Autodesk Inventor part; units mm, degrees
ref_plane "YZ Plane" through (0, 0, 0) normal (1, 0, 0) x (0, 1, 0)
ref_plane "XZ Plane" through (0, 0, 0) normal (0, 1, 0) x (-1, 0, 0)
ref_plane "XY Plane" through (0, 0, 0) normal (0, 0, 1) x (1, 0, 0)
sketch "Sketch1" plane through (0, 0, 0) normal (0, 0, 1) x (1, 0, 0)
  line L0 (-25.4, -12.7) -> (25.4, -12.7)
  line L1 (25.4, -12.7) -> (25.4, 12.7)
  line L2 (25.4, 12.7) -> (-25.4, 12.7)
  line L3 (-25.4, 12.7) -> (-25.4, -12.7)
  line L4 (-25.4, -12.7) -> (25.4, 12.7) construction
  line L5 (25.4, -12.7) -> (-25.4, 12.7) construction
  line L6 (-22.225, -9.525) -> (22.225, -9.525)
  line L7 (22.225, -9.525) -> (22.225, 9.525)
  line L8 (22.225, 9.525) -> (-22.225, 9.525)
  line L9 (-22.225, 9.525) -> (-22.225, -9.525)
  line L10 (-22.225, -9.525) -> (22.225, 9.525) construction
  line L11 (22.225, -9.525) -> (-22.225, 9.525) construction
  line L12 (0, 9.525) -> (0, 12.7) construction
  line L13 (22.225, 0) -> (25.4, 0) construction
  point P0 (0, 0)
  dimension "d0" = 25.4
  dimension "d1" = 50.8
  dimension "d2" = 3.175
extrude "Extrusion1" add sketch "Sketch1" along normal blind 488.95
sketch "Sketch2" plane through (-25.4, 12.7, 0) normal (0, 1, 0) x (1, 0, 0)
  circle A0 centre (19.05, -469.9) radius 11.1125
  circle A1 centre (31.75, -256.8674) radius 11.1125
  circle A2 centre (25.4, -363.3837) radius 11.1125
  circle A3 centre (15.875, -19.05) radius 11.1125
  line L0 (0, 0) -> (0, -488.95) construction
  line L1 (3.175, 0) -> (3.175, -488.95) construction
  line L2 (50.8, 0) -> (50.8, -488.95) construction
  line L3 (15.875, -19.05) -> (24.1367, -26.4818) construction
  line L4 (19.05, -469.9) -> (31.75, -256.8674) construction
  line L5 (50.8, -488.95) -> (0, -488.95)
  line L6 (47.625, 0) -> (47.625, -488.95) construction
  circle A4 centre (38.1, -237.8174) radius 1.905
  circle A5 centre (38.1, -275.9174) radius 1.905
  circle A6 centre (9.525, -256.8674) radius 1.905
  line L7 (38.1, -237.8174) -> (38.1, -275.9174) construction
  line L8 (9.525, -256.8674) -> (47.625, -256.8674) construction
  circle A7 centre (31.75, -256.8674) radius 14.2875 construction
  circle A8 centre (19.05, -469.9) radius 14.2875 construction
  circle A9 centre (31.75, -256.8674) radius 14.2875 construction
  circle A10 centre (15.875, -19.05) radius 14.2875 construction
  point P0 (25.4, -363.3837)
  point P1 (38.1, -256.8674)
  dimension "d10" = 22.225
  dimension "d5" = 22.225
  dimension "d16" = 19.05
  dimension "d17" = 19.05
  dimension "d20" = 19.05
  dimension "d21" = 15.875
  dimension "d23" = 19.05
  dimension "d24" = 38.1
  dimension "d27" = 28.575
  dimension "d28" = 3.81
  dimension "d29" = 22.225
  dimension "d31" = 106.7054
  dimension "d32" = 28.575
  dimension "d34" = 6.35
extrude "Extrusion2" cut sketch "Sketch2" against normal through all
fillet "Fillet1" radius 19.05 3 edges at (-25.4, 0, 0) (-25.4, 0, 488.95) (25.4, 0, 488.95)
properties part number "arm" material "Aluminum 6061"
Can you work these out from the model? Positions are in its coordinate system, mm. A direction names the side the tool comes from. Give positions to 0.01 mm unless a question says otherwise; leave off trailing zeros. Loops run counter-clockwise (first coordinate to the right, second up) from the corner with the lowest first, then second, coordinate; pieces in that order, holes last. Notation, with made-up numbers: M 14.25,-19 L 55.25,-19 A10 ccw 55.25,-3 Z; hole C -30.5,-26.75 d5. An arc over 180 degrees is marked long. Use one line per item in the form item = value. Start each with the question number.
(1) Thinking about a two-plate mould opening in X: for faces 3 (the cylindrical face through (-23.526, 0.178, 10.81)), 4 (the cylindrical face through (-10.97, -11.09, 8.03)), 5 (the cylindrical face through (23.703, -0.178, 477.761)), which applies, released by +X, released by -X, zero draft, split by the parting line, or undercut?
(2) I want a section at A-A, the plane z = 437. Write out the boundary of the cut face in (x, y) (3 decimals).
(3) On a 3-axis mill with a long thin cutter (end or side, diameter ignored), from which of +Z, -Z, +X, -X, +Y, -Y can I reach the whole of each face in a straight line? I mean faces 1 (the cylindrical face through (-10.97, 11.13, 8.03)), 2 (the flat face through (22.225, 0, 237)). Say none if no direction works.
(4) Please list where these lines run through material, in increasing order: line 1 (Y direction, x = 14.5, z = 281) (3 decimals); line 2 (Z direction, x = 6.35, y = -10.6); line 3 (Z direction, x = 5, y = 10.5).
Worked out:
q1.face_3 = released by -X
q1.face_4 = undercut
q1.face_5 = released by +X
q2.outline = M -25.4,-12.7 L 25.4,-12.7 L 25.4,12.7 L -25.4,12.7 Z; hole M -22.225,-9.525 L 22.225,-9.525 L 22.225,9.525 L -22.225,9.525 Z
q3.face_1 = +Y, -Y
q3.face_2 = +Z, -Z
q4.line_1 = -12.7 to -9.525, 9.525 to 12.7
q4.line_2 = 0 to 245.75, 267.98 to 354.26, 372.5 to 488.95
q4.line_3 = 0 to 245.84, 267.9 to 353.46, 373.31 to 488.95
